from build123d import *

# Parameters (mm, degrees)
TUBO_RETANGULAR_50_X_30_X_2_6_1_DEPTH = 689.8
ESBO_O5_R                             = 3
CORTE_EXTRUS_O4_DEPTH                 = 692.772390313
ESBO_O6_R                             = 3.5
CORTE_EXTRUS_O5_DEPTH                 = 692.772390313


with BuildPart() as part:
    # Sketch1 → Tubo retangular 50 X 30 X 2.6(1) (new body)
    with BuildSketch(Plane.YZ):
        with BuildLine():
            Line((-12, -25), (12, -25))
            ThreePointArc((12, -25), (14.121320344, -24.121320344), (15, -22))
            Line((15, -22), (15, 22))
            ThreePointArc((15, 22), (14.121320344, 24.121320344), (12, 25))
            Line((12, 25), (-12, 25))
            ThreePointArc((-12, 25), (-14.121320344, 24.121320344), (-15, 22))
            Line((-15, 22), (-15, -22))
            ThreePointArc((-15, -22), (-14.121320344, -24.121320344), (-12, -25))
        make_face()
        with BuildLine():
            Line((-12, -23.8), (12, -23.8))
            ThreePointArc((12, -23.8), (13.272792206, -23.272792206), (13.8, -22))
            Line((13.8, -22), (13.8, 22))
            ThreePointArc((13.8, 22), (13.272792206, 23.272792206), (12, 23.8))
            Line((12, 23.8), (-12, 23.8))
            ThreePointArc((-12, 23.8), (-13.272792206, 23.272792206), (-13.8, 22))
            Line((-13.8, 22), (-13.8, -22))
            ThreePointArc((-13.8, -22), (-13.272792206, -23.272792206), (-12, -23.8))
        make_face(mode=Mode.SUBTRACT)
    extrude(amount=TUBO_RETANGULAR_50_X_30_X_2_6_1_DEPTH)

    # Esboço5 → Corte-extrusão4 (cut, through all)
    with BuildSketch(Plane.XY.offset(25)):
        with Locations((280.1625, -0.6530272)):
            Circle(ESBO_O5_R)
        with Locations((240.1625, -0.6530272)):
            Circle(ESBO_O5_R)
        with Locations((595.6625, -0.6530272)):
            Circle(ESBO_O5_R)
        with Locations((555.6625, -0.6530272)):
            Circle(ESBO_O5_R)
    extrude(amount=-CORTE_EXTRUS_O4_DEPTH, mode=Mode.SUBTRACT)

    # Esboço6 → Corte-extrusão5 (cut, through all)
    with BuildSketch(Plane.XY.offset(25)):
        with Locations((102, 1.769410095)):
            Circle(ESBO_O6_R)
    extrude(amount=-CORTE_EXTRUS_O5_DEPTH, mode=Mode.SUBTRACT)


solid = part.part
Source: CAD feature listing. Evaluate the final solid. Frame: model axes, mm. A direction names the side the tool comes from. Coordinates: 2 decimals unless noted, no trailing zeros. Write each loop counter-clockwise with the first axis right and the second up, starting at its lowest first coordinate (ties: lowest second). Pieces come first, ordered by that corner, then holes. Notation, with made-up numbers: M 50.25,16 L 81.25,16 A23 ccw 81.25,44 Z; hole C 27.25,13.25 d2. An arc over 180 degrees is marked long. Use a Markdown table: item, result.
1) Section B-B, the plane z = -13. Output: boundary loops of the cut face in (x, y), then the cut area to 3 significant figures.
Conclusion:
| item | result |
|---|---|
| outline | M 0,-15 L 689.8,-15 L 689.8,-13.8 L 0,-13.8 Z; M 0,13.8 L 689.8,13.8 L 689.8,15 L 0,15 Z |
| area | 1,660 mm^2 |
2) Mould query, pull axis Y, two halves, no side actions, for faces 1 (the flat face through (340, 0, -23.8)), 2 (the flat face through (340, 0, -25)), 3 (the flat face through (340, 0, 23.8)), 4 (the flat face through (340, -15, 0)). Classes: pulls with the +Y half, pulls with the -Y half, needs draft (parallel to the pull), parting line crosses it, or undercut.
Conclusion:
| item | result |
|---|---|
| face 1 | undercut |
| face 2 | needs draft |
| face 3 | undercut |
| face 4 | pulls with the -Y half |
3) Reachability of faces 5 (the flat face through (340, 0, 25)), 6 (the flat face through (340, 13.8, 0)) from +Z, -Z, +X, -X, +Y, -Y: full face, straight path, thin tool, end or side. Return the list, or none.
Conclusion:
| item | result |
|---|---|
| face 5 | +Z, +X, -X, +Y, -Y |
| face 6 | +X, -X |
4) First-contact query: pin 1 Ø5.5 at (x, y) = (240.16, -0.65) entering from +Z; pin 2 Ø7 at (x, y) = (595.66, -0.65) entering from -Z. Flat tips, straight axial feed; report the tip coordinate or a pass-through.
Conclusion:
| item | result |
|---|---|
| pin 1 | passes through |
| pin 2 | stops at z = -25 |
5) Ray query, L1, parallel to Z at x = 402, y = -11; L2, parallel to Y at x = 438.5, z = 9; L3, parallel to Y at x = 102, z = 24. Return the intervals inside material, ascending.
Conclusion:
| item | result |
|---|---|
| L1 | z = -25 to -23.8, 23.8 to 25 |
| L2 | y = -15 to -13.8, 13.8 to 15 |
| L3 | y = -14.24 to -1.73, 5.27 to 14.24 |
6) Section A-A, the plane x = 172.5. Output: boundary loops of the cut face in (y, z), then the cut area to 3 significant figures.
Conclusion:
| item | result |
|---|---|
| outline | M -15,-22 A3 ccw -12,-25 L 12,-25 A3 ccw 15,-22 L 15,22 A3 ccw 12,25 L -12,25 A3 ccw -15,22 Z; hole M -13.8,-22 A1.8 ccw -12,-23.8 L 12,-23.8 A1.8 ccw 13.8,-22 L 13.8,22 A1.8 ccw 12,23.8 L -12,23.8 A1.8 ccw -13.8,22 Z |
| area | 181 mm^2 |
